Here's how the part is built. I have some questions about the finished solid (model axes, mm). A direction names the side the tool comes from. Round coordinates to 2 decimals unless told otherwise and drop trailing zeros. Write each loop counter-clockwise with the first axis right and the second up, starting at its lowest first coordinate (ties: lowest second). Pieces come first, ordered by that corner, then holes. Notation, with made-up numbers: (9, -2.5) -> (55, -2.5) arc R14 cw to (55, 20.5) -> close; hole circle Ø6 at (68, 40.5). An arc over 180 degrees is marked (long way). Answer as CSV lines item,"result".
```python
from build123d import *

# Parameters (mm, degrees)
F0_R              = 35
F0_R_2            = 33
F2_DEPTH          = 31
F3_DEPTH          = 18
F4_E28_W          = 6
F4_E28_H          = 7.5
F4_E39_MIRRORCS_W = 6
F4_E39_MIRRORCS_H = 7.5
F5_DEPTH          = 9.3
F7_DEPTH          = 4
F8_R              = 21.1
F9_R              = 2
F10_DEPTH         = 38
F11_DEPTH         = 52
F12_DEPTH         = 37.9
F13_R             = 33.8752288108
F14_DEPTH         = 4.9
F15_W             = 4.2938441038
F15_H             = 3.1884626523
F16_DEPTH         = 17.2


with BuildPart() as f2:
    # F0 (on Top) → F2 (new body)
    with BuildSketch(Plane.XY):
        Circle(F0_R)
        Circle(F0_R_2, mode=Mode.SUBTRACT)
    extrude(amount=F2_DEPTH)

    # F1 (on Top) → F3 (join)
    with BuildSketch(Plane.XY):
        Polygon((10, -32.0528298616), (10, -24), (10, 32.2797112167), (6, 33.4707275033), (6, 12), (3, 12), (0, 12), (-3, 12), (-6, 12), (-6, 33.4707275033), (-10, 32.2797112167), (-10, -24), (-10, -32.0528298616), (-6, -33.1044308841), (-6, -24), (0, -24), (6, -24), (6, -33.1044308841), align=None)
        Polygon((0, 7), (3, 7), (3, 5), (6, 5), (6, -19), (0, -19), (-6, -19), (-6, 5), (-3, 5), (-3, 7), align=None, mode=Mode.SUBTRACT)
    extrude(amount=F3_DEPTH)

    # F4_E28 (on explicit) + F4_E39_MirrorCS (on explicit) → F5 (cut)
    with BuildSketch(Plane.XZ.offset(24)):
        with Locations((3, 3.75)):
            Rectangle(F4_E28_W, F4_E28_H)
    with BuildSketch(Plane(origin=(0, -24, 0), x_dir=(-1, 0, 0), z_dir=(0, 1, 0))):
        with Locations((3, 3.75)):
            Rectangle(F4_E39_MIRRORCS_W, F4_E39_MIRRORCS_H)
    extrude(amount=-F5_DEPTH, dir=(0, -1, 0), mode=Mode.SUBTRACT)

    # F6 (on Top) → F7 (join)
    with BuildSketch(Plane.XY):
        Polygon((60.8495350583, 35.131495446), (-60.8495350583, 35.131495446), (0, -70.2629908919), align=None)
    extrude(amount=F7_DEPTH)

    # F8
    f8_edges = [f2.edges().sort_by_distance(p)[0] for p in [
        (-60.849535, 35.131495, 2),
        (60.849535, 35.131495, 2),
        (0, -70.262991, 2),
    ]]
    fillet(f8_edges, radius=F8_R)

    # F9 (on Top) → F10 (cut)
    with BuildSketch(Plane.XY):
        with Locations((-37.2817739844, 20.93468979)):
            Circle(F9_R)
        with Locations((0, -42.7055284381)):
            Circle(F9_R)
        with Locations((36.2159647048, 19.8873784393)):
            Circle(F9_R)
    extrude(amount=-F10_DEPTH, mode=Mode.SUBTRACT)

    # F9 (on Top) → F11 (cut)
    with BuildSketch(Plane.XY):
        with Locations((36.2159647048, 19.8873784393)):
            Circle(F9_R)
    extrude(amount=F11_DEPTH, mode=Mode.SUBTRACT)

    # F9 (on Top) → F12 (cut)
    with BuildSketch(Plane.XY):
        with Locations((-37.2817739844, 20.93468979)):
            Circle(F9_R)
        with Locations((0, -42.7055284381)):
            Circle(F9_R)
    extrude(amount=F12_DEPTH, mode=Mode.SUBTRACT)

    # F13 (on Top) → F14 (cut)
    with BuildSketch(Plane.XY):
        Circle(F13_R)
    extrude(amount=F14_DEPTH, mode=Mode.SUBTRACT)

    # F15 (on face) → F16 (cut)
    with BuildSketch(Plane(origin=(0, 35.131495446, 0), x_dir=(-1, 0, 0), z_dir=(0, 1, 0))):
        Polygon((-7.865479216, 7.1884626523), (-0.6682581179, 7.1884626523), (0.0053993426, 7.1884626523), (0.0053993426, 10.3769253045), (4.2992434464, 10.3769253045), (4.2992434464, 7.1884626523), (7.865479216, 7.1884626523), (7.865479216, 11.9928242639), (-7.865479216, 11.9928242639), align=None)
        with Locations((2.1523213945, 8.7826939784)):
            Rectangle(F15_W, F15_H)
        with Locations((2.1523213945, 5.5942313261)):
            Rectangle(F15_W, F15_H)
    extrude(amount=-F16_DEPTH, mode=Mode.SUBTRACT)


solid = f2.part
```
1. Suppose I cut it at C-C on z = 26.5. Please give me the cut outline in (x, y).
Numbers:
outline,"circle Ø70 at (0, 0); hole circle Ø66 at (0, 0)"
2. Suppose I cut it at D-D on x = 21.5. Please give me the cut outline in (y, z).
Numbers:
outline,"(-33.02, 0) -> (-26.18, 0) -> (-26.18, 4.9) -> (-25.03, 4.9) -> (-25.03, 31) -> (-27.62, 31) -> (-27.62, 4) -> (-33.02, 4) -> close; (25.03, 4.9) -> (26.18, 4.9) -> (26.18, 0) -> (35.13, 0) -> (35.13, 4) -> (27.62, 4) -> (27.62, 31) -> (25.03, 31) -> close"
3. If I drill on line 1 (Y direction, x = 0, z = 23.75); line 2 (X direction, y = 10.5, z = 9.5); line 3 (X direction, y = -17, z = 17), over which ranges is the centre line in solid material (lowest first)?
Numbers:
line 1,"y = -35 to -33, 33 to 35"
line 2,"x = -33.39 to -31.28, -10 to 10, 31.28 to 33.39"
line 3,"x = -30.59 to -28.28, -10 to -6, 6 to 10, 28.28 to 30.59"
4. If we mould it in two halves opening along Y, with no side actions, what happens to faces 4 (the face through (7, 0, 18)), 5 (the face through (0, 35.131, 2)), 6 (the face through (-42.42, 24.85, 2.03)), 7 (the face through (-4.299, 34, 6))? For each: released by +Y, released by -Y, zero draft, split by the parting line, or undercut.
Numbers:
face 4,"undercut"
face 5,"released by +Y"
face 6,"split by the parting line"
face 7,"zero draft"
5. For pin 1 Ø3 at (y, z) = (-15.5, 3.5) entering from -X; pin 2 Ø12 at (x, y) = (-17.5, -3.5) entering from +Z; pin 3 Ø8 at (x, z) = (-22, 26) entering from -Y; pin 4 Ø0.9 at (x, z) = (4, 12.5) entering from -Y, each with a flat end and sliding along its axis, tell me the tip position at first contact or that it passes through.
Numbers:
pin 1,"stops at x = -32.48"
pin 2,"passes through"
pin 3,"stops at y = -30.02"
pin 4,"stops at y = -34.82"
6. Suppose I cut it at A-A on y = -10. Please give me the cut outline in (x, z).
Numbers:
outline,"(-34.79, 0) -> (-32.37, 0) -> (-32.37, 4.9) -> (-31.45, 4.9) -> (-31.45, 31) -> (-33.54, 31) -> (-33.54, 4) -> (-34.79, 4) -> close; (-10, 4.9) -> (-6, 4.9) -> (-6, 18) -> (-10, 18) -> close; (6, 4.9) -> (10, 4.9) -> (10, 18) -> (6, 18) -> close; (31.45, 4.9) -> (32.37, 4.9) -> (32.37, 0) -> (34.79, 0) -> (34.79, 4) -> (33.54, 4) -> (33.54, 31) -> (31.45, 31) -> close"
7. Suppose I cut it at B-B on x = -26. Please give me the cut outline in (y, z).
Numbers:
outline,"(-25.23, 0) -> (-21.71, 0) -> (-21.71, 4.9) -> (-20.32, 4.9) -> (-20.32, 31) -> (-23.43, 31) -> (-23.43, 4) -> (-25.23, 4) -> close; (20.32, 4.9) -> (21.71, 4.9) -> (21.71, 0) -> (35.06, 0) -> (35.06, 4) -> (23.43, 4) -> (23.43, 31) -> (20.32, 31) -> close"
8. On a 3-axis mill with a long thin cutter (end or side, diameter ignored), from which of +Z, -Z, +X, -X, +Y, -Y can I reach the whole of each face in a straight line? I mean faces 1 (the face through (6.3, 28.4, 7.188)), 2 (the face through (3, 6, 11)), 3 (the face through (30.255, -17.86, 1.972)). Say none if no direction works.
Numbers:
face 1,"+Y"
face 2,"+Z, -Z"
face 3,"+Z, -Z, +X, -Y"
